from build123d import *

# Parameters (mm, degrees)
F1_DEPTH = 1.8
F2_R     = 0.6
F3_SIZE2 = 0.5494954839
F3_SIZE  = 0.2


with BuildPart() as f1:
    # F0 (on Top) → F1 (new body)
    with BuildSketch(Plane.XY):
        with BuildLine():
            Line((29.9906235347, 0.75), (28.4901298698, 0.75))
            ThreePointArc((28.4901298698, 0.75), (28.4975323606, 0.3750324718), (28.5, 0))
            ThreePointArc((28.5, 0), (28.4975323606, -0.3750324718), (28.4901298698, -0.75))
            Line((28.4901298698, -0.75), (29.9906235347, -0.75))
            Line((29.9906235347, -0.75), (29.9906235347, 0.75))
        make_face()
        with BuildLine():
            Line((21.2132034356, 21.2132034356), (20.1525432638, 20.1525432638))
            ThreePointArc((20.1525432638, 20.1525432638), (26.1847681615, 11.2520183224), (28.4901298698, 0.75))
            Line((28.4901298698, 0.75), (29.9906235347, 0.75))
            ThreePointArc((29.9906235347, 0.75), (27.570702708, 11.8260877803), (21.2132034356, 21.2132034356))
        make_face()
        with BuildLine():
            Line((28.4901298698, 0.75), (5.4486236794, 0.75))
            ThreePointArc((5.4486236794, 0.75), (5.4871408874, 0.3758788124), (5.5, 0))
            ThreePointArc((5.5, 0), (5.4871408874, -0.3758788124), (5.4486236794, -0.75))
            Line((5.4486236794, -0.75), (28.4901298698, -0.75))
            ThreePointArc((28.4901298698, -0.75), (28.4975323606, -0.3750324718), (28.5, 0))
            ThreePointArc((28.5, 0), (28.4975323606, 0.3750324718), (28.4901298698, 0.75))
        make_face()
        with BuildLine():
            ThreePointArc((28.4901298698, -0.75), (26.1847681615, -11.2520183224), (20.1525432638, -20.1525432638))
            Line((20.1525432638, -20.1525432638), (21.2132034356, -21.2132034356))
            ThreePointArc((21.2132034356, -21.2132034356), (27.570702708, -11.8260877803), (29.9906235347, -0.75))
            Line((29.9906235347, -0.75), (28.4901298698, -0.75))
        make_face()
        with BuildLine():
            ThreePointArc((3.1224989992, 2.5), (3.7742546282, 1.3247648854), (4, 0))
            ThreePointArc((4, 0), (3.7742546282, -1.3247648854), (3.1224989992, -2.5))
            ThreePointArc((3.1224989992, -2.5), (2.979991028, -2.6682678787), (2.8284271247, -2.8284271247))
            Line((2.8284271247, -2.8284271247), (3.8890872965, -3.8890872965))
            ThreePointArc((3.8890872965, -3.8890872965), (4.9256145638, -2.4471046501), (5.4486236794, -0.75))
            Line((5.4486236794, -0.75), (5.4486236794, 0.75))
            ThreePointArc((5.4486236794, 0.75), (4.9256145638, 2.4471046501), (3.8890872965, 3.8890872965))
            Line((3.8890872965, 3.8890872965), (2.8284271247, 2.8284271247))
            ThreePointArc((2.8284271247, 2.8284271247), (2.979991028, 2.6682678787), (3.1224989992, 2.5))
        make_face()
        with BuildLine():
            ThreePointArc((3.1224989992, -2.5), (3.7742546282, -1.3247648854), (4, 0))
            ThreePointArc((4, 0), (3.7742546282, 1.3247648854), (3.1224989992, 2.5))
            Line((3.1224989992, 2.5), (2.5370304368, 2.03125))
            ThreePointArc((2.5370304368, 2.03125), (3.0665818854, 1.0763714694), (3.25, 0))
            ThreePointArc((3.25, 0), (3.0665818854, -1.0763714694), (2.5370304368, -2.03125))
            Line((2.5370304368, -2.03125), (3.1224989992, -2.5))
        make_face()
        with BuildLine():
            Line((-0.2, 3.2438403167), (-0.2, 3.9949968711))
            ThreePointArc((-0.2, 3.9949968711), (-4, 0), (-0.2, -3.9949968711))
            Line((-0.2, -3.9949968711), (-0.2, -3.2438403167))
            ThreePointArc((-0.2, -3.2438403167), (-3.25, 0), (-0.2, 3.2438403167))
        make_face()
        with BuildLine():
            ThreePointArc((-0.2, 3.9949968711), (1.4378381449, 3.7326426924), (2.8284271247, 2.8284271247))
            Line((2.8284271247, 2.8284271247), (3.8890872965, 3.8890872965))
            ThreePointArc((3.8890872965, 3.8890872965), (-5.5, 0), (3.8890872965, -3.8890872965))
            Line((3.8890872965, -3.8890872965), (2.8284271247, -2.8284271247))
            ThreePointArc((2.8284271247, -2.8284271247), (1.4378381449, -3.7326426924), (-0.2, -3.9949968711))
            ThreePointArc((-0.2, -3.9949968711), (-4, 0), (-0.2, 3.9949968711))
        make_face()
        with BuildLine():
            ThreePointArc((5.5, 0), (5.4871408874, 0.3758788124), (5.4486236794, 0.75))
            Line((5.4486236794, 0.75), (5.4486236794, -0.75))
            ThreePointArc((5.4486236794, -0.75), (5.4871408874, -0.3758788124), (5.5, 0))
        make_face()
        with BuildLine():
            ThreePointArc((30, 0), (29.9976557921, 0.3750293049), (29.9906235347, 0.75))
            Line((29.9906235347, 0.75), (29.9906235347, -0.75))
            ThreePointArc((29.9906235347, -0.75), (29.9976557921, -0.3750293049), (30, 0))
        make_face()
    extrude(amount=F1_DEPTH)

    # F2
    f2_edges = [f1.edges().sort_by_distance(p)[0] for p in [
        (21.213203, -21.213203, 0.9),
        (20.152543, -20.152543, 0.9),
        (21.213203, 21.213203, 0.9),
        (20.152543, 20.152543, 0.9),
    ]]
    fillet(f2_edges, radius=F2_R)

    # F3
    f3_edges = [f1.edges().sort_by_distance(p)[0] for p in [
        (-3.25, 0, 0),
        (-0.2, 3.619419, 0),
        (1.641342, 3.647738, 0),
        (3.25, 0, 0),
        (2.829765, 2.265625, 0),
        (2.829765, -2.265625, 0),
        (1.641342, -3.647738, 0),
        (-0.2, -3.619419, 0),
    ]]
    f3_side = f1.faces().sort_by_distance((14.942774, 0, 0))[0]
    chamfer(f3_edges, length=F3_SIZE, length2=F3_SIZE2, reference=f3_side)


solid = f1.part
Build history of the part. All positions in model axes, mm. A direction names the side the tool comes from. Give positions to 0.01 mm unless a question says otherwise; leave off trailing zeros. Order: outer loops, then holes, each group sorted by start corner. A loop starts at its lowest first (then second) coordinate and runs counter-clockwise, first axis right, second up. Notation, with made-up numbers: M 4,54 L 12,54 A10 ccw 12,67 Z; hole C 77.25,21.25 d3. An arc over 180 degrees is marked long. Use one line per item in the form item = value.
Q1. Pin check, flat tips, straight feed: P1, Ø1, axis at x = 6.5, z = 1.5, coming from the -Y side; P2, Ø0.8, axis at y = -3.5, z = 1, coming from the +X side. Stop position of each tip, or through.
Conclusion:
P1 = -0.75
P2 = 29.84
Q2. Slice it at B-B, the plane x = 23. Write the cut outline in (y, z), and give its area (3 significant figures).
Conclusion:
outline = M -19.26,0 L -16.83,0 L -16.83,1.8 L -19.26,1.8 Z; M -0.75,0 L 0.75,0 L 0.75,1.8 L -0.75,1.8 Z; M 16.83,0 L 19.26,0 L 19.26,1.8 L 16.83,1.8 Z
area = 11.5 mm2
Q3. Pull direction Y, two halves, no side cores. Call faces 4 (the cylindrical face through (21.21, -20.96, 0.91)), 5 (the cylindrical face through (26.24, 11.12, 0.89)), 6 (the cylindrical face through (20.4, 20.2, 0.9)), 7 (the cylindrical face through (21.22, 20.96, 0.91)): released by +Y, released by -Y, zero draft, split by the parting line, or undercut.
Conclusion:
face_4 = released by -Y
face_5 = undercut
face_6 = undercut
face_7 = released by +Y
Q4. Wall check: probe 1 along Y at (x, z) = (21, 1.35); probe 2 along Y at (x, z) = (11, 0.7); probe 3 along Y at (x, z) = (-2, 0.6). Give the ranges that are in metal, low to high.
Conclusion:
probe_1 = -20.92 to -19.27, -0.75 to 0.75, 19.27 to 20.92
probe_2 = -0.75 to 0.75
probe_3 = -5.12 to -2.56, 2.56 to 5.12
Q5. Slice it at D-D, the plane y = -7. Write the cut outline in (x, z).
Conclusion:
outline = M 27.63,0 L 29.17,0 L 29.17,1.8 L 27.63,1.8 Z
Q6. Slice it at C-C, the plane x = 17.5. Write the cut outline in (y, z), and give its area (3 significant figures).
Conclusion:
outline = M -0.75,0 L 0.75,0 L 0.75,1.8 L -0.75,1.8 Z
area = 2.70 mm2
Q7. Which spindle directions (+Z, -Z, +X, -X, +Y, -Y) get a long thin tool onto all of the face, cutting with end or side? Do faces 1 (the cylindrical face through (20.4, -20.1, 0.9)), 2 (the conical face through (-3.303, -0.07, 0.401)), 3 (the flat face through (17, -0.75, 1)). Say none if no direction does.
Conclusion:
face_1 = +Z, -Z, -X
face_2 = -Z
face_3 = +Z, -Z
